Can you work these out from the model? Positions are in its coordinate system, mm. Give positions to 0.01 mm unless a question says otherwise; leave off trailing zeros. Answer as a JSON object with one key per item and string values.
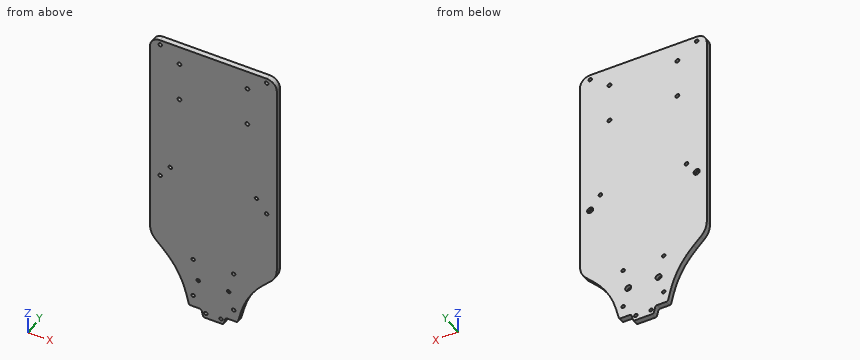
```python
from build123d import *

# Parameters (mm, degrees)
DECK_BASE_DEPTH       = 5.5
BOLT_SLOT_REACH       = 7.5
SKETCH_3_R            = 1.75
SKETCH_14_R           = 3
BOLT_HEAD_DEPTH       = 2
FILLET_1_R            = 4
CUT_EXTRUDE_6_REACH   = 7.5
SKETCH_15_W           = 145
SKETCH_15_H           = 39
CUT_EXTRUDE_7_DEPTH   = 10
FILLET_2_R            = 2
SKETCH_17_OUTSIDE_W   = 211.856
SKETCH_17_OUTSIDE_H   = 356.856
SKETCH_17_OUTSIDE_W_2 = 125
SKETCH_17_OUTSIDE_H_2 = 290
CUT_EXTRUDE_8_DEPTH   = 10
FILLET_4_R            = 10
FILLET_5_R            = 20
LIDAR_SLOT_REACH      = 7.5
SKETCH_4_R            = 1.7
VESC_SLOT_REACH       = 7.5
SKETCH_6_R            = 1.9
NANO_SLOT_REACH       = 7.5
SKETCH_7_R            = 1.75
CUT_EXTRUDE_3_REACH   = 7.5
SKETCH_12_R           = 1.75
SKETCH_13_R           = 3
CUT_EXTRUDE_4_DEPTH   = 3.7


with BuildPart() as part:
    # 스케치1 → Deck base (new body)
    with BuildSketch(Plane(origin=(0, 0, 0), x_dir=(1, 0, 0), z_dir=(0, 1, 0))):
        with BuildLine():
            Line((-72.5, 0), (-72.5, -185))
            ThreePointArc((-72.5, -185), (-69.571067812, -192.071067812), (-62.5, -195))
            Line((-62.5, -195), (-49.962007487, -195))
            ThreePointArc((-49.962007487, -195), (-47.753248675, -195.514313374), (-45.998887542, -196.951446196))
            Line((-45.998887542, -196.951446196), (-19.001112458, -232.048553804))
            ThreePointArc((-19.001112458, -232.048553804), (-17.246751325, -233.485686626), (-15.037992513, -234))
            Line((-15.037992513, -234), (15.037992513, -234))
            ThreePointArc((15.037992513, -234), (17.246751325, -233.485686626), (19.001112458, -232.048553804))
            Line((19.001112458, -232.048553804), (45.998887542, -196.951446196))
            ThreePointArc((45.998887542, -196.951446196), (47.753248675, -195.514313374), (49.962007487, -195))
            Line((49.962007487, -195), (62.5, -195))
            ThreePointArc((62.5, -195), (69.571067812, -192.071067812), (72.5, -185))
            Line((72.5, -185), (72.5, 0))
            ThreePointArc((72.5, 0), (70.204904333, 11.508182998), (63.670781605, 21.255540601))
            Line((63.670781605, 21.255540601), (49.478231298, 35.391496426))
            ThreePointArc((49.478231298, 35.391496426), (35.536990456, 53.662264501), (27, 75))
            Line((27, 75), (22, 95))
            Line((22, 95), (-22, 95))
            Line((-22, 95), (-27, 75))
            ThreePointArc((-27, 75), (-35.536990456, 53.662264501), (-49.478231298, 35.391496426))
            Line((-49.478231298, 35.391496426), (-63.670781605, 21.255540601))
            ThreePointArc((-63.670781605, 21.255540601), (-70.204904333, 11.508182998), (-72.5, 0))
        make_face()
    extrude(amount=DECK_BASE_DEPTH)

    # 스케치3 → Bolt slot (cut, up to next)
    with BuildSketch(Plane(origin=(0, 5.5, 0), x_dir=(1, 0, 0), z_dir=(0, 1, 0)), mode=Mode.PRIVATE) as bolt_slot_sk1:
        with Locations((7.5, 90)):
            Circle(SKETCH_3_R)
    bolt_slot_tool1 = extrude(bolt_slot_sk1.sketch, amount=-BOLT_SLOT_REACH, mode=Mode.PRIVATE) & part.part
    add(bolt_slot_tool1.solids().sort_by_distance((7.5, 5.5, -90))[0], mode=Mode.SUBTRACT)
    # 스케치3 → Bolt slot (cut, up to next)
    with BuildSketch(Plane(origin=(0, 5.5, 0), x_dir=(1, 0, 0), z_dir=(0, 1, 0)), mode=Mode.PRIVATE) as bolt_slot_sk2:
        with Locations((-7.5, 90)):
            Circle(SKETCH_3_R)
    bolt_slot_tool2 = extrude(bolt_slot_sk2.sketch, amount=-BOLT_SLOT_REACH, mode=Mode.PRIVATE) & part.part
    add(bolt_slot_tool2.solids().sort_by_distance((-7.5, 5.5, -90))[0], mode=Mode.SUBTRACT)
    # 스케치3 → Bolt slot (cut, up to next)
    with BuildSketch(Plane(origin=(0, 5.5, 0), x_dir=(1, 0, 0), z_dir=(0, 1, 0)), mode=Mode.PRIVATE) as bolt_slot_sk3:
        with Locations((52.5, -45)):
            Circle(SKETCH_3_R)
    bolt_slot_tool3 = extrude(bolt_slot_sk3.sketch, amount=-BOLT_SLOT_REACH, mode=Mode.PRIVATE) & part.part
    add(bolt_slot_tool3.solids().sort_by_distance((52.5, 5.5, 45))[0], mode=Mode.SUBTRACT)
    # 스케치3 → Bolt slot (cut, up to next)
    with BuildSketch(Plane(origin=(0, 5.5, 0), x_dir=(1, 0, 0), z_dir=(0, 1, 0)), mode=Mode.PRIVATE) as bolt_slot_sk4:
        with Locations((52.5, -190)):
            Circle(SKETCH_3_R)
    bolt_slot_tool4 = extrude(bolt_slot_sk4.sketch, amount=-BOLT_SLOT_REACH, mode=Mode.PRIVATE) & part.part
    add(bolt_slot_tool4.solids().sort_by_distance((52.5, 5.5, 190))[0], mode=Mode.SUBTRACT)
    # 스케치3 → Bolt slot (cut, up to next)
    with BuildSketch(Plane(origin=(0, 5.5, 0), x_dir=(1, 0, 0), z_dir=(0, 1, 0)), mode=Mode.PRIVATE) as bolt_slot_sk5:
        with Locations((-52.5, -190)):
            Circle(SKETCH_3_R)
    bolt_slot_tool5 = extrude(bolt_slot_sk5.sketch, amount=-BOLT_SLOT_REACH, mode=Mode.PRIVATE) & part.part
    add(bolt_slot_tool5.solids().sort_by_distance((-52.5, 5.5, 190))[0], mode=Mode.SUBTRACT)
    # 스케치3 → Bolt slot (cut, up to next)
    with BuildSketch(Plane(origin=(0, 5.5, 0), x_dir=(1, 0, 0), z_dir=(0, 1, 0)), mode=Mode.PRIVATE) as bolt_slot_sk6:
        with Locations((-52.5, -45)):
            Circle(SKETCH_3_R)
    bolt_slot_tool6 = extrude(bolt_slot_sk6.sketch, amount=-BOLT_SLOT_REACH, mode=Mode.PRIVATE) & part.part
    add(bolt_slot_tool6.solids().sort_by_distance((-52.5, 5.5, 45))[0], mode=Mode.SUBTRACT)

    # 스케치14 → Bolt head (cut)
    with BuildSketch(Plane(origin=(0, 5.5, 0), x_dir=(1, 0, 0), z_dir=(0, 1, 0))):
        with Locations((-52.5, -45)):
            Circle(SKETCH_14_R)
        with Locations((52.5, -45)):
            Circle(SKETCH_14_R)
    extrude(amount=-BOLT_HEAD_DEPTH, mode=Mode.SUBTRACT)

    # 필렛1
    fillet_1_edges = [part.edges().sort_by_distance(p)[0] for p in [
        (22, 2.75, -95),
        (-22, 2.75, -95),
    ]]
    fillet(fillet_1_edges, radius=FILLET_1_R)

    # 스케치15 → 컷-돌출6 (cut, up to next)
    with BuildSketch(Plane(origin=(0, 5.5, 0), x_dir=(1, 0, 0), z_dir=(0, 1, 0)), mode=Mode.PRIVATE) as cut_extrude_6_sk1:
        with Locations((0, -214.5)):
            Rectangle(SKETCH_15_W, SKETCH_15_H)
    cut_extrude_6_tool1 = extrude(cut_extrude_6_sk1.sketch, amount=-CUT_EXTRUDE_6_REACH, mode=Mode.PRIVATE) & part.part
    add(cut_extrude_6_tool1.solids().sort_by_distance((0, 5.5, 214.5))[0], mode=Mode.SUBTRACT)

    # 스케치16 → 컷-돌출7 (cut)
    with BuildSketch(Plane(origin=(0, 5.5, 0), x_dir=(1, 0, 0), z_dir=(0, 1, 0))):
        Polygon((-9.999999999, 95), (10.000000001, 95), (12.000000001, 87), (24, 87), (24, 100), (-24, 100), (-24, 87), (-11.999999999, 87), align=None)
    extrude(amount=-CUT_EXTRUDE_7_DEPTH, mode=Mode.SUBTRACT)

    # 필렛2
    fillet_2_edges = [part.edges().sort_by_distance(p)[0] for p in [
        (-9.999999999, 2.75, -95),
        (-11.999999999, 2.75, -87),
        (-24, 2.75, -87),
        (24, 2.75, -87),
        (12.000000001, 2.75, -87),
        (10.000000001, 2.75, -95),
    ]]
    fillet(fillet_2_edges, radius=FILLET_2_R)

    # 스케치17 outside → 컷-돌출8 (cut)
    with BuildSketch(Plane(origin=(0, 5.5, 0), x_dir=(1, 0, 0), z_dir=(0, 1, 0))):
        with Locations((0, -50)):
            Rectangle(SKETCH_17_OUTSIDE_W, SKETCH_17_OUTSIDE_H)
        with Locations((0, -50)):
            Rectangle(SKETCH_17_OUTSIDE_W_2, SKETCH_17_OUTSIDE_H_2, mode=Mode.SUBTRACT)
    extrude(amount=-CUT_EXTRUDE_8_DEPTH, mode=Mode.SUBTRACT)

    # 필렛4
    fillet_4_edges = [part.edges().sort_by_distance(p)[0] for p in [
        (-62.5, 2.75, 195),
        (62.5, 2.75, 195),
    ]]
    fillet(fillet_4_edges, radius=FILLET_4_R)

    # 필렛5
    fillet_5_edges = [part.edges().sort_by_distance(p)[0] for p in [
        (-62.5, 2.75, -22.421653575),
        (62.5, 2.75, -22.421653575),
    ]]
    fillet(fillet_5_edges, radius=FILLET_5_R)

    # 스케치4 → Lidar slot (cut, up to next)
    with BuildSketch(Plane(origin=(0, 5.5, 0), x_dir=(1, 0, 0), z_dir=(0, 1, 0)), mode=Mode.PRIVATE) as lidar_slot_sk1:
        with Locations((-20, 75)):
            Circle(SKETCH_4_R)
    lidar_slot_tool1 = extrude(lidar_slot_sk1.sketch, amount=-LIDAR_SLOT_REACH, mode=Mode.PRIVATE) & part.part
    add(lidar_slot_tool1.solids().sort_by_distance((-20, 5.5, -75))[0], mode=Mode.SUBTRACT)
    # 스케치4 → Lidar slot (cut, up to next)
    with BuildSketch(Plane(origin=(0, 5.5, 0), x_dir=(1, 0, 0), z_dir=(0, 1, 0)), mode=Mode.PRIVATE) as lidar_slot_sk2:
        with Locations((-20, 35)):
            Circle(SKETCH_4_R)
    lidar_slot_tool2 = extrude(lidar_slot_sk2.sketch, amount=-LIDAR_SLOT_REACH, mode=Mode.PRIVATE) & part.part
    add(lidar_slot_tool2.solids().sort_by_distance((-20, 5.5, -35))[0], mode=Mode.SUBTRACT)
    # 스케치4 → Lidar slot (cut, up to next)
    with BuildSketch(Plane(origin=(0, 5.5, 0), x_dir=(1, 0, 0), z_dir=(0, 1, 0)), mode=Mode.PRIVATE) as lidar_slot_sk3:
        with Locations((20, 35)):
            Circle(SKETCH_4_R)
    lidar_slot_tool3 = extrude(lidar_slot_sk3.sketch, amount=-LIDAR_SLOT_REACH, mode=Mode.PRIVATE) & part.part
    add(lidar_slot_tool3.solids().sort_by_distance((20, 5.5, -35))[0], mode=Mode.SUBTRACT)
    # 스케치4 → Lidar slot (cut, up to next)
    with BuildSketch(Plane(origin=(0, 5.5, 0), x_dir=(1, 0, 0), z_dir=(0, 1, 0)), mode=Mode.PRIVATE) as lidar_slot_sk4:
        with Locations((20, 75)):
            Circle(SKETCH_4_R)
    lidar_slot_tool4 = extrude(lidar_slot_sk4.sketch, amount=-LIDAR_SLOT_REACH, mode=Mode.PRIVATE) & part.part
    add(lidar_slot_tool4.solids().sort_by_distance((20, 5.5, -75))[0], mode=Mode.SUBTRACT)

    # 스케치6 → Vesc slot (cut, up to next)
    with BuildSketch(Plane(origin=(0, 5.5, 0), x_dir=(1, 0, 0), z_dir=(0, 1, 0)), mode=Mode.PRIVATE) as vesc_slot_sk1:
        with Locations((33.5, -137)):
            Circle(SKETCH_6_R)
    vesc_slot_tool1 = extrude(vesc_slot_sk1.sketch, amount=-VESC_SLOT_REACH, mode=Mode.PRIVATE) & part.part
    add(vesc_slot_tool1.solids().sort_by_distance((33.5, 5.5, 137))[0], mode=Mode.SUBTRACT)
    # 스케치6 → Vesc slot (cut, up to next)
    with BuildSketch(Plane(origin=(0, 5.5, 0), x_dir=(1, 0, 0), z_dir=(0, 1, 0)), mode=Mode.PRIVATE) as vesc_slot_sk2:
        with Locations((33.5, -176)):
            Circle(SKETCH_6_R)
    vesc_slot_tool2 = extrude(vesc_slot_sk2.sketch, amount=-VESC_SLOT_REACH, mode=Mode.PRIVATE) & part.part
    add(vesc_slot_tool2.solids().sort_by_distance((33.5, 5.5, 176))[0], mode=Mode.SUBTRACT)
    # 스케치6 → Vesc slot (cut, up to next)
    with BuildSketch(Plane(origin=(0, 5.5, 0), x_dir=(1, 0, 0), z_dir=(0, 1, 0)), mode=Mode.PRIVATE) as vesc_slot_sk3:
        with Locations((-33.5, -176)):
            Circle(SKETCH_6_R)
    vesc_slot_tool3 = extrude(vesc_slot_sk3.sketch, amount=-VESC_SLOT_REACH, mode=Mode.PRIVATE) & part.part
    add(vesc_slot_tool3.solids().sort_by_distance((-33.5, 5.5, 176))[0], mode=Mode.SUBTRACT)
    # 스케치6 → Vesc slot (cut, up to next)
    with BuildSketch(Plane(origin=(0, 5.5, 0), x_dir=(1, 0, 0), z_dir=(0, 1, 0)), mode=Mode.PRIVATE) as vesc_slot_sk4:
        with Locations((-33.5, -137)):
            Circle(SKETCH_6_R)
    vesc_slot_tool4 = extrude(vesc_slot_sk4.sketch, amount=-VESC_SLOT_REACH, mode=Mode.PRIVATE) & part.part
    add(vesc_slot_tool4.solids().sort_by_distance((-33.5, 5.5, 137))[0], mode=Mode.SUBTRACT)

    # 스케치7 → Nano slot (cut, up to next)
    with BuildSketch(Plane(origin=(0, 5.5, 0), x_dir=(1, 0, 0), z_dir=(0, 1, 0)), mode=Mode.PRIVATE) as nano_slot_sk1:
        with Locations((-42.5, -58)):
            Circle(SKETCH_7_R)
    nano_slot_tool1 = extrude(nano_slot_sk1.sketch, amount=-NANO_SLOT_REACH, mode=Mode.PRIVATE) & part.part
    add(nano_slot_tool1.solids().sort_by_distance((-42.5, 5.5, 58))[0], mode=Mode.SUBTRACT)
    # 스케치7 → Nano slot (cut, up to next)
    with BuildSketch(Plane(origin=(0, 5.5, 0), x_dir=(1, 0, 0), z_dir=(0, 1, 0)), mode=Mode.PRIVATE) as nano_slot_sk2:
        with Locations((42.5, -58)):
            Circle(SKETCH_7_R)
    nano_slot_tool2 = extrude(nano_slot_sk2.sketch, amount=-NANO_SLOT_REACH, mode=Mode.PRIVATE) & part.part
    add(nano_slot_tool2.solids().sort_by_distance((42.5, 5.5, 58))[0], mode=Mode.SUBTRACT)

    # 스케치12 → 컷-돌출3 (cut, up to next)
    with BuildSketch(Plane(origin=(0, 5.5, 0), x_dir=(1, 0, 0), z_dir=(0, 1, 0)), mode=Mode.PRIVATE) as cut_extrude_3_sk1:
        with Locations((-15, 56.5)):
            Circle(SKETCH_12_R)
    cut_extrude_3_tool1 = extrude(cut_extrude_3_sk1.sketch, amount=-CUT_EXTRUDE_3_REACH, mode=Mode.PRIVATE) & part.part
    add(cut_extrude_3_tool1.solids().sort_by_distance((-15, 5.5, -56.5))[0], mode=Mode.SUBTRACT)
    # 스케치12 → 컷-돌출3 (cut, up to next)
    with BuildSketch(Plane(origin=(0, 5.5, 0), x_dir=(1, 0, 0), z_dir=(0, 1, 0)), mode=Mode.PRIVATE) as cut_extrude_3_sk2:
        with Locations((15, 56.5)):
            Circle(SKETCH_12_R)
    cut_extrude_3_tool2 = extrude(cut_extrude_3_sk2.sketch, amount=-CUT_EXTRUDE_3_REACH, mode=Mode.PRIVATE) & part.part
    add(cut_extrude_3_tool2.solids().sort_by_distance((15, 5.5, -56.5))[0], mode=Mode.SUBTRACT)

    # 스케치13 → 컷-돌출4 (cut)
    with BuildSketch(Plane(origin=(0, 5.5, 0), x_dir=(1, 0, 0), z_dir=(0, 1, 0))):
        with Locations((-15, 56.5)):
            Circle(SKETCH_13_R)
        with Locations((15, 56.5)):
            Circle(SKETCH_13_R)
    extrude(amount=-CUT_EXTRUDE_4_DEPTH, mode=Mode.SUBTRACT)


solid = part.part
```
1) I need wall thicknesses on L1, parallel to Z at x = 20, y = 1.9; L2, parallel to X at y = 2.5, z = 45; L3, parallel to Z at x = -33.5, y = 1.25. Which ranges of each line are inside material? Lowest first, please.
Results found:
{"L1": "z = -87 to -76.7, -73.3 to -36.7, -33.3 to 195", "L2": "x = -62.5 to -54.25, -50.75 to 50.75, 54.25 to 62.5", "L3": "z = -57.47 to 135.1, 138.9 to 174.1, 177.9 to 195"}
2) I want a section at A-A on y = 4.35. Count the separate pieces of the cut face and the enclosed holes in it, and give its area (3 significant figures).
Results found:
{"separate pieces": "1", "enclosed holes": "18", "area": "31,900 mm²"}
3) I'm going to push flat-ended pins straight in: pin 1 Ø6 at (x, z) = (33.5, 137) entering from -Y; pin 2 Ø3 at (x, z) = (15, -56.5) entering from +Y; pin 3 Ø3 at (x, z) = (15.5, -56.5) entering from +Y. Where does each tip first touch, or does it pass through?
Results found:
{"pin 1": "stops at y = 0", "pin 2": "passes through", "pin 3": "stops at y = 1.8"}
